Design review of the part built by this model. Coordinates are the model's own, in mm. A direction names the side the tool comes from. Coordinates: 2 decimals unless noted, no trailing zeros. Loops run counter-clockwise (first coordinate to the right, second up) from the corner with the lowest first, then second, coordinate; pieces in that order, holes last. Notation, with made-up numbers: (21.25, -39) - (32.25, -39) arc R22 cw to (32.25, -21) - close; hole circle Ø10 at (52, 8.5). An arc over 180 degrees is marked (long way). Answer in a Markdown table with one row per item. Add a question column.
(1) To check wall thickness, follow L1, parallel to X at y = -9.5, z = 3.6; L2, parallel to Y at x = -15.5, z = 2.05; L3, parallel to Y at x = -29.5, z = 0.95. State the ranges of each line that lie inside material, in increasing order. Write a range as [from, to].
(2) We need section C-C, the plane x = 28. Write out the cut boundary in (y, z).
(3) The part is to be moulded in two halves that separate along X. For faces 5 (the face through (35.73, -39.11, 1.97)), 6 (the face through (15.726, 30.845, 1.972)), 7 (the face through (-18.072, -9, 2)), 8 (the face through (-35.73, -39.08, 1.97)), say which applies: released by +X, released by -X, zero draft, split by the parting line, or undercut.
(4) Clearance check with flat-ended pins moving along their axes: pin 1 (6.5 mm diameter, centred on x = 28.49, y = -36.48, fed in from -Z); pin 2 (1.5 mm diameter, centred on y = -0.5, z = 2, fed in from +X); pin 3 (2 mm diameter, centred on y = 24.5, z = 1, fed in from -X); pin 4 (1.2 mm diameter, centred on y = -1, z = 1.5, fed in from -X). State where each tip first meets the part, or that it passes through.
(5) For faces 1 (the face through (-5.536, 30.676, 1.972)), 2 (the face through (11, 23, 2)), 3 (the face through (20.367, -3, 2)), 4 (the face through (-20.538, -16.064, 1.972)), list the 3-axis set-ups (+Z, -Z, +X, -X, +Y, -Y) from which the entire face can be reached by the end or side of a thin tool; tool diameter is ignored.
(6) We need section A-A, the plane y = -10.5. Write out the cut boundary in (x, z), plus the area to 3 significant figures.
(7) We need section B-B, the plane x = 15. Write out the cut boundary in (y, z).
(8) We need section D-D, the plane z = 2.3. Give the number of separate pieces and of enclosed holes in the cut face, plus the area to 3 significant figures.
from build123d import *

# Parameters (mm, degrees)
F0_R     = 2.05
F0_R_2   = 1.55
F1_DEPTH = 4


with BuildPart() as f1:
    # F0 (on Top) → F1 (new body)
    with BuildSketch(Plane.XY):
        with BuildLine():
            ThreePointArc((20.225759, -40.726859), (20.88342, -41.207836), (21.646246, -41.494115))
            Line((21.646246, -41.494115), (25.044904, -42.264138))
            Line((25.044904, -42.264138), (30.325992, -43.460657))
            ThreePointArc((30.325992, -43.460657), (31.363938, -43.61615), (32.391927, -43.404607))
            ThreePointArc((32.391927, -43.404607), (34.248228, -42.031919), (35.554256, -40.128129))
            ThreePointArc((35.554256, -40.128129), (35.729228, -39.093288), (35.537043, -38.061505))
            Line((35.537043, -38.061505), (34.154086, -32.826147))
            Line((34.154086, -32.826147), (33.264079, -29.456918))
            ThreePointArc((33.264079, -29.456918), (32.950942, -28.704719), (32.446956, -28.06452))
            Line((32.446956, -28.06452), (21.831277, -17.818679))
            Line((21.831277, -17.818679), (21.048334, -16.865171))
            ThreePointArc((21.048334, -16.865171), (20.542366, -15.972423), (20.366866, -14.961383))
            Line((20.366866, -14.961383), (20.366866, 9.177489))
            ThreePointArc((20.366866, 9.177489), (20.542466, 10.188808), (21.04871, 11.081736))
            ThreePointArc((21.04871, 11.081736), (21.427756, 11.516935), (21.831277, 11.929542))
            Line((21.831277, 11.929542), (32.446956, 22.175383))
            ThreePointArc((32.446956, 22.175383), (32.950942, 22.815582), (33.264079, 23.567781))
            Line((33.264079, 23.567781), (34.154086, 26.93701))
            Line((34.154086, 26.93701), (35.537043, 32.172368))
            ThreePointArc((35.537043, 32.172368), (35.729228, 33.204151), (35.554256, 34.238992))
            ThreePointArc((35.554256, 34.238992), (34.248228, 36.142781), (32.391927, 37.515469))
            ThreePointArc((32.391927, 37.515469), (31.363938, 37.727013), (30.325992, 37.57152))
            Line((30.325992, 37.57152), (25.044904, 36.375001))
            Line((25.044904, 36.375001), (21.646246, 35.604977))
            ThreePointArc((21.646246, 35.604977), (20.88342, 35.318699), (20.225759, 34.837722))
            Line((20.225759, 34.837722), (19.467341, 34.105726))
            Line((19.467341, 34.105726), (17.506323, 32.213028))
            ThreePointArc((17.506323, 32.213028), (15.698461, 30.828478), (13.62424, 29.888823))
            ThreePointArc((13.62424, 29.888823), (11.43078, 29.508538), (9.217452, 29.74742))
            Line((9.217452, 29.74742), (1.956759, 31.578982))
            ThreePointArc((1.956759, 31.578982), (0, 31.821979), (-1.956759, 31.578982))
            Line((-1.956759, 31.578982), (-9.217452, 29.74742))
            ThreePointArc((-9.217452, 29.74742), (-11.43078, 29.508538), (-13.62424, 29.888823))
            ThreePointArc((-13.62424, 29.888823), (-15.698461, 30.828478), (-17.506323, 32.213028))
            Line((-17.506323, 32.213028), (-19.467341, 34.105726))
            Line((-19.467341, 34.105726), (-20.225759, 34.837722))
            ThreePointArc((-20.225759, 34.837722), (-20.88342, 35.318699), (-21.646246, 35.604977))
            Line((-21.646246, 35.604977), (-25.044904, 36.375001))
            Line((-25.044904, 36.375001), (-30.325992, 37.57152))
            ThreePointArc((-30.325992, 37.57152), (-31.363938, 37.727013), (-32.391927, 37.515469))
            ThreePointArc((-32.391927, 37.515469), (-34.248228, 36.142781), (-35.554256, 34.238992))
            ThreePointArc((-35.554256, 34.238992), (-35.729228, 33.204151), (-35.537043, 32.172368))
            Line((-35.537043, 32.172368), (-34.154086, 26.93701))
            Line((-34.154086, 26.93701), (-33.264079, 23.567781))
            ThreePointArc((-33.264079, 23.567781), (-32.950942, 22.815582), (-32.446956, 22.175383))
            Line((-32.446956, 22.175383), (-21.831277, 11.929542))
            ThreePointArc((-21.831277, 11.929542), (-21.427756, 11.516935), (-21.04871, 11.081736))
            ThreePointArc((-21.04871, 11.081736), (-20.542466, 10.188808), (-20.366866, 9.177489))
            Line((-20.366866, 9.177489), (-20.366866, -15.066626))
            ThreePointArc((-20.366866, -15.066626), (-20.542466, -16.077945), (-21.04871, -16.970873))
            ThreePointArc((-21.04871, -16.970873), (-21.427756, -17.406072), (-21.831277, -17.818679))
            Line((-21.831277, -17.818679), (-32.446956, -28.06452))
            ThreePointArc((-32.446956, -28.06452), (-32.950942, -28.704719), (-33.264079, -29.456918))
            Line((-33.264079, -29.456918), (-34.154086, -32.826147))
            Line((-34.154086, -32.826147), (-35.537043, -38.061505))
            ThreePointArc((-35.537043, -38.061505), (-35.729228, -39.093288), (-35.554256, -40.128129))
            ThreePointArc((-35.554256, -40.128129), (-34.248228, -42.031919), (-32.391927, -43.404607))
            ThreePointArc((-32.391927, -43.404607), (-31.363938, -43.61615), (-30.325992, -43.460657))
            Line((-30.325992, -43.460657), (-25.044904, -42.264138))
            Line((-25.044904, -42.264138), (-21.646246, -41.494115))
            ThreePointArc((-21.646246, -41.494115), (-20.88342, -41.207836), (-20.225759, -40.726859))
            Line((-20.225759, -40.726859), (-19.467341, -39.994863))
            Line((-19.467341, -39.994863), (-17.506323, -38.102165))
            ThreePointArc((-17.506323, -38.102165), (-14.306504, -36.02511), (-10.561704, -35.29746))
            Line((-10.561704, -35.29746), (10.561704, -35.29746))
            ThreePointArc((10.561704, -35.29746), (14.306504, -36.02511), (17.506323, -38.102165))
            Line((17.506323, -38.102165), (19.467341, -39.994863))
            Line((19.467341, -39.994863), (20.225759, -40.726859))
        make_face()
        with Locations((-28.491992, -36.476224)):
            Circle(F0_R, mode=Mode.SUBTRACT)
        with Locations((-22.735756, -30.920528)):
            Circle(F0_R, mode=Mode.SUBTRACT)
        with Locations((-15.321724, -28.768979)):
            Circle(F0_R_2, mode=Mode.SUBTRACT)
        with BuildLine():
            ThreePointArc((-16.233353, -16.307766), (-16.438378, -16.802741), (-16.933353, -17.007766))
            Line((-16.933353, -17.007766), (-17.371724, -17.007766))
            ThreePointArc((-17.371724, -17.007766), (-17.866699, -16.802741), (-18.071724, -16.307766))
            Line((-18.071724, -16.307766), (-18.071724, -1.707766))
            ThreePointArc((-18.071724, -1.707766), (-17.866699, -1.212792), (-17.371724, -1.007766))
            Line((-17.371724, -1.007766), (-16.933353, -1.007766))
            ThreePointArc((-16.933353, -1.007766), (-16.438378, -1.212792), (-16.233353, -1.707766))
            Line((-16.233353, -1.707766), (-16.233353, -16.307766))
        make_face(mode=Mode.SUBTRACT)
        with Locations((15.178276, -28.768979)):
            Circle(F0_R_2, mode=Mode.SUBTRACT)
        with Locations((28.491992, -36.476224)):
            Circle(F0_R, mode=Mode.SUBTRACT)
        with Locations((22.735756, -30.920528)):
            Circle(F0_R, mode=Mode.SUBTRACT)
        with BuildLine():
            Line((17.371724, -17.007766), (16.933353, -17.007766))
            ThreePointArc((16.933353, -17.007766), (16.438378, -16.802741), (16.233353, -16.307766))
            Line((16.233353, -16.307766), (16.233353, -1.707766))
            ThreePointArc((16.233353, -1.707766), (16.438378, -1.212792), (16.933353, -1.007766))
            Line((16.933353, -1.007766), (17.371724, -1.007766))
            ThreePointArc((17.371724, -1.007766), (17.866699, -1.212792), (18.071724, -1.707766))
            Line((18.071724, -1.707766), (18.071724, -16.307766))
            ThreePointArc((18.071724, -16.307766), (17.866699, -16.802741), (17.371724, -17.007766))
        make_face(mode=Mode.SUBTRACT)
        with Locations((-15.321724, 1.731021)):
            Circle(F0_R_2, mode=Mode.SUBTRACT)
        with Locations((-22.735756, 25.031391)):
            Circle(F0_R, mode=Mode.SUBTRACT)
        with Locations((-28.491992, 30.587086)):
            Circle(F0_R, mode=Mode.SUBTRACT)
        with BuildLine():
            Line((-10.6, 27.367114), (-9.9, 27.367114))
            ThreePointArc((-9.9, 27.367114), (-9.617157, 27.249957), (-9.5, 26.967114))
            Line((-9.5, 26.967114), (-9.5, 19.739609))
            ThreePointArc((-9.5, 19.739609), (-9.617157, 19.456766), (-9.9, 19.339609))
            Line((-9.9, 19.339609), (-10.6, 19.339609))
            ThreePointArc((-10.6, 19.339609), (-10.882843, 19.456766), (-11, 19.739609))
            Line((-11, 19.739609), (-11, 26.967114))
            ThreePointArc((-11, 26.967114), (-10.882843, 27.249957), (-10.6, 27.367114))
        make_face(mode=Mode.SUBTRACT)
        with Locations((15.178276, 1.731021)):
            Circle(F0_R_2, mode=Mode.SUBTRACT)
        with BuildLine():
            Line((9.5, 24.008841), (9.5, 26.967114))
            ThreePointArc((9.5, 26.967114), (9.617157, 27.249957), (9.9, 27.367114))
            Line((9.9, 27.367114), (10.6, 27.367114))
            ThreePointArc((10.6, 27.367114), (10.882843, 27.249957), (11, 26.967114))
            Line((11, 26.967114), (11, 19.739609))
            ThreePointArc((11, 19.739609), (10.882843, 19.456766), (10.6, 19.339609))
            Line((10.6, 19.339609), (9.9, 19.339609))
            ThreePointArc((9.9, 19.339609), (9.617157, 19.456766), (9.5, 19.739609))
            Line((9.5, 19.739609), (9.5, 24.008841))
        make_face(mode=Mode.SUBTRACT)
        with Locations((22.735756, 25.031391)):
            Circle(F0_R, mode=Mode.SUBTRACT)
        with Locations((28.491992, 30.587086)):
            Circle(F0_R, mode=Mode.SUBTRACT)
    extrude(amount=F1_DEPTH)


solid = f1.part
Responses:
| question | item | result |
|---|---|---|
| 1 | L1 | x = [-20.37, -18.07], [-16.23, 16.23], [18.07, 20.37] |
| 1 | L2 | y = [-36.6, -30.31], [-27.23, 0.19], [3.27, 30.71] |
| 1 | L3 | y = [-43.27, -38.26], [-34.69, -25.22], [19.33, 28.8], [32.37, 37.38] |
| 2 | outline | (-42.93, 0) - (-38.47, 0) - (-38.47, 4) - (-42.93, 4) - close; (-34.49, 0) - (-23.77, 0) - (-23.77, 4) - (-34.49, 4) - close; (17.88, 0) - (28.6, 0) - (28.6, 4) - (17.88, 4) - close; (32.58, 0) - (37.04, 0) - (37.04, 4) - (32.58, 4) - close |
| 3 | face 5 | released by +X |
| 3 | face 6 | undercut |
| 3 | face 7 | undercut |
| 3 | face 8 | released by -X |
| 4 | pin 1 | stops at z = 0 |
| 4 | pin 2 | stops at x = 20.37 |
| 4 | pin 3 | stops at x = -33.77 |
| 4 | pin 4 | stops at x = -20.37 |
| 5 | face 1 | +Z, -Z, +Y |
| 5 | face 2 | +Z, -Z |
| 5 | face 3 | +Z, -Z, +X |
| 5 | face 4 | +Z, -Z, -X |
| 6 | outline | (-20.37, 0) - (-18.07, 0) - (-18.07, 4) - (-20.37, 4) - close; (-16.23, 0) - (16.23, 0) - (16.23, 4) - (-16.23, 4) - close; (18.07, 0) - (20.37, 0) - (20.37, 4) - (18.07, 4) - close |
| 6 | area | 148 mm2 |
| 7 | outline | (-36.34, 0) - (-30.31, 0) - (-30.31, 4) - (-36.34, 4) - close; (-27.23, 0) - (0.19, 0) - (0.19, 4) - (-27.23, 4) - close; (3.27, 0) - (30.45, 0) - (30.45, 4) - (3.27, 4) - close |
| 8 | separate pieces | 1 |
| 8 | enclosed holes | 16 |
| 8 | area | 3,620 mm2 |
